```python
from build123d import *

# Parameters (mm, degrees)
SKETCH1_W           = 47
SKETCH1_H           = 60
BOSS_EXTRUDE1_DEPTH = 20
SHELL1_T            = -5
FILLET2_R           = 2
FILLET3_R           = 2
FILLET4_R           = 2
FILLET5_R           = 2
FILLET6_R           = 2
FILLET7_R           = 2
FILLET8_R           = 2
FILLET9_R           = 2
FILLET10_R          = 2
SKETCH2_R           = 2
CUT_EXTRUDE1_DEPTH  = 10


with BuildPart() as part:
    # Sketch1 → Boss-Extrude1 (new body)
    with BuildSketch(Plane(origin=(0, 0, 0), x_dir=(1, 0, 0), z_dir=(0, 1, 0))):
        with Locations((2.676470588, -4.572192513)):
            Rectangle(SKETCH1_W, SKETCH1_H)
    extrude(amount=BOSS_EXTRUDE1_DEPTH)

    # Shell1
    shell1_openings = [part.faces().sort_by_distance(p)[0] for p in [
        (2.676470588, 20, 4.572192513),
    ]]
    offset(amount=SHELL1_T, openings=shell1_openings, kind=Kind.INTERSECTION)

    # Fillet2
    fillet2_edges = [part.edges().sort_by_distance(p)[0] for p in [
        (21.176470588, 12.5, 29.572192513),
    ]]
    fillet(fillet2_edges, radius=FILLET2_R)

    # Fillet3
    fillet3_edges = [part.edges().sort_by_distance(p)[0] for p in [
        (-15.823529412, 12.5, 29.572192513),
    ]]
    fillet(fillet3_edges, radius=FILLET3_R)

    # Fillet4
    fillet4_edges = [part.edges().sort_by_distance(p)[0] for p in [
        (-15.823529412, 12.5, -20.427807487),
    ]]
    fillet(fillet4_edges, radius=FILLET4_R)

    # Fillet5
    fillet5_edges = [part.edges().sort_by_distance(p)[0] for p in [
        (21.176470588, 12.5, -20.427807487),
    ]]
    fillet(fillet5_edges, radius=FILLET5_R)

    # Fillet6
    fillet6_edges = [part.edges().sort_by_distance(p)[0] for p in [
        (-20.823529412, 10, 34.572192513),
    ]]
    fillet(fillet6_edges, radius=FILLET6_R)

    # Fillet7
    fillet7_edges = [part.edges().sort_by_distance(p)[0] for p in [
        (26.176470588, 10, 34.572192513),
    ]]
    fillet(fillet7_edges, radius=FILLET7_R)

    # Fillet8
    fillet8_edges = [part.edges().sort_by_distance(p)[0] for p in [
        (-20.823529412, 10, -25.427807487),
    ]]
    fillet(fillet8_edges, radius=FILLET8_R)

    # Fillet9
    fillet9_edges = [part.edges().sort_by_distance(p)[0] for p in [
        (26.176470588, 10, -25.427807487),
    ]]
    fillet(fillet9_edges, radius=FILLET9_R)

    # Fillet10
    fillet10_edges = [part.edges().sort_by_distance(p)[0] for p in [
        (2.676470588, 0, 34.572192513),
        (26.176470588, 0, 4.572192513),
        (-20.823529412, 0, 4.572192513),
        (2.676470588, 0, -25.427807487),
    ]]
    fillet(fillet10_edges, radius=FILLET10_R)

    # Sketch2 → Cut-Extrude1 (cut)
    with BuildSketch(Plane(origin=(0, 0, 0), x_dir=(1, 0, 0), z_dir=(0, 1, 0))):
        with Locations((-6.280636193, 7.634914268)):
            Circle(SKETCH2_R)
        with Locations((2.676470588, -4.572192513)):
            Circle(SKETCH2_R)
        with Locations((11.633577369, -16.779299295)):
            Circle(SKETCH2_R)
    extrude(amount=CUT_EXTRUDE1_DEPTH, mode=Mode.SUBTRACT)


solid = part.part
```
Model file for the job. Use its own axes, mm. A direction names the side the tool comes from. Round coordinates to 2 decimals unless told otherwise and drop trailing zeros. Write each loop counter-clockwise with the first axis right and the second up, starting at its lowest first coordinate (ties: lowest second). Pieces come first, ordered by that corner, then holes. Notation, with made-up numbers: M -20.5,10.5 L -4.5,10.5 A19 ccw -4.5,17.5 Z; hole C 2.5,71 d8. An arc over 180 degrees is marked long. Put each result on its own line as item: value.
Item 1: Flat gauge pins, fed straight in: P1, Ø3.5, axis at x = 11.63, z = 16.78, coming from the +Y side; P2, Ø18.5, axis at x = 8.5, z = 4, coming from the +Y side. Where does each tip first touch, or does it go through?
Responses:
P1: through
P2: y = 5
Item 2: Probe L1, parallel to Z at x = 1, y = 12.5; L2, parallel to X at y = 11.5, z = 11.5; L3, parallel to Y at x = 4, z = -5. List the from-to ranges inside material, lowest first. Write a range as from..to.
Responses:
L1: -25.43..-20.43, 29.57..34.57
L2: -20.82..-15.82, 21.18..26.18
L3: 0..5
Item 3: Cut at C-C (z = 1.5). List the corners of the cut face in (x, y), and give its area (3 significant figures).
Responses:
outline: M -20.82,2 A2 ccw -18.82,0 L 24.18,0 A2 ccw 26.18,2 L 26.18,20 L 21.18,20 L 21.18,5 L -15.82,5 L -15.82,20 L -20.82,20 Z
area: 383 mm²
Item 4: Cut at D-D (x = -10). List the corners of the cut face in (y, z), and give its area (3 significant figures).
Responses:
outline: M 0,-23.43 A2 ccw 2,-25.43 L 20,-25.43 L 20,-20.43 L 5,-20.43 L 5,29.57 L 20,29.57 L 20,34.57 L 2,34.57 A2 ccw 0,32.57 Z
area: 448 mm²
Item 5: Cut at B-B (x = -5). List the corners of the cut face in (y, z), and give its area (3 significant figures).
Responses:
outline: M 0,-23.43 A2 ccw 2,-25.43 L 20,-25.43 L 20,-20.43 L 5,-20.43 L 5,-9.17 L 0,-9.17 Z; M 0,-6.1 L 5,-6.1 L 5,29.57 L 20,29.57 L 20,34.57 L 2,34.57 A2 ccw 0,32.57 Z
area: 433 mm²
Item 6: Mould opens along X. For faces 3 (the cylindrical face through (3, 0.6, 34)), 4 (the flat face through (26.176, 11, 5)), 5 (the cylindrical face through (-8.28, 2.46, -7.72)) say: +X half, -X half, draft (parallel to the pull), parting line (faces both ways), or undercut.
Responses:
face 3: draft
face 4: +X half
face 5: undercut
Item 7: Cut at A-A (y = 6.25). List the corners of the cut face in (x, z), and give its area (3 significant figures).
Responses:
outline: M -20.82,-23.43 A2 ccw -18.82,-25.43 L 24.18,-25.43 A2 ccw 26.18,-23.43 L 26.18,32.57 A2 ccw 24.18,34.57 L -18.82,34.57 A2 ccw -20.82,32.57 Z; hole M -15.82,-18.43 A2 ccw -13.82,-20.43 L 19.18,-20.43 A2 ccw 21.18,-18.43 L 21.18,27.57 A2 ccw 19.18,29.57 L -13.82,29.57 A2 ccw -15.82,27.57 Z
area: 970 mm²
Item 8: Tool access for faces 1 (the flat face through (2, 12, -20.428)), 2 (the flat face through (-2, 0, 4)): list every direction of +Z, -Z, +X, -X, +Y, -Y with a clear straight run to the whole face (end or side of a thin tool).
Responses:
face 1: +Y
face 2: +Z, -Z, +X, -X, -Y
